Geometry: final body of the model. Coordinates: model frame, mm. A direction names the side the tool comes from. Give positions to 0.01 mm unless a question says otherwise; leave off trailing zeros. Write each loop counter-clockwise with the first axis right and the second up, starting at its lowest first coordinate (ties: lowest second). Pieces come first, ordered by that corner, then holes. Notation, with made-up numbers: (11, 27.25) - (18, 27.25) arc R25 cw to (18, 64.25) - close; hole circle Ø11 at (88, 84). An arc over 180 degrees is marked (long way). Return JSON: item names as keys, results as strings.
Autodesk Inventor part; units mm, degrees
ref_plane "YZ Plane" through (0, 0, 0) normal (1, 0, 0) x (0, 1, 0)
ref_plane "XZ Plane" through (0, 0, 0) normal (0, 1, 0) x (-1, 0, 0)
ref_plane "XY Plane" through (0, 0, 0) normal (0, 0, 1) x (1, 0, 0)
sketch "Sketch1" plane through (0, 0, 0) normal (0, 1, 0) x (-1, 0, 0)
  line L0 (1100, 990) -> (-1100, 990)
  line L1 (-1100, 990) -> (-1100, 0)
  line L2 (-1100, 0) -> (1100, 0)
  line L3 (1100, 0) -> (1100, 990)
  point P0 (0, 0)
  point P1 (0, 0)
  dimension "d0" = 2200
  dimension "d1" = 990
extrude "Extrusion1" add sketch "Sketch1" along normal blind 1020
sketch "Sketch2" plane through (1100, 0, 990) normal (1, 0, 0) x (0, 0, -1)
  line L0 (0, 0) -> (0, 1020)
  line L1 (0, 1020) -> (740, 1020)
  line L2 (740, 1020) -> (740, 600)
  line L3 (740, 600) -> (0, 600)
  line L4 (0, 600) -> (0, 1020)
  line L5 (990, 0) -> (990, 1020)
  point P0 (0, 600)
  dimension "d4" = 600
  dimension "d5" = 250
extrude "Extrusion2" cut sketch "Sketch2" against normal through all
sketch "Sketch3" plane through (1100, 600, 990) normal (0, 1, 0) x (1, 0, 0)
  line L0 (-2200, 0) -> (0, 0)
  line L1 (-2200, 740) -> (0, 740)
  line L2 (-1950, 0) -> (-250, 0)
  line L3 (-250, 0) -> (-250, 740)
  line L4 (-250, 740) -> (-1950, 740)
  line L5 (-1950, 740) -> (-1950, 0)
  line L6 (-2200, 0) -> (-2200, 740)
  point P0 (-1100, 990)
  point P1 (-1100, 0)
  point P2 (-1100, 0)
  point P3 (-1950, 740)
  point P4 (-250, 0)
  dimension "d8" = 250
extrude "Extrusion3" cut sketch "Sketch3" against normal blind 250 contours L5 L1 L3 L0
sketch "Sketch4" plane through (0, 0, 0) normal (0, -1, 0) x (1, 0, 0)
  line L0 (1100, 990) -> (1100, 0)
  line L1 (-1100, 990) -> (1100, 990)
  line L2 (-1100, 0) -> (-1100, 990)
  line L3 (1100, 0) -> (-1100, 0)
  line L4 (1000, 890) -> (1000, 100) construction
  line L5 (1000, 100) -> (-1000, 100) construction
  line L6 (-1000, 100) -> (-1000, 890) construction
  line L7 (-1000, 890) -> (1000, 890) construction
  circle A0 centre (-1000, 890) radius 25
  circle A1 centre (1000, 890) radius 25
  circle A2 centre (1000, 100) radius 25
  circle A3 centre (-1000, 100) radius 25
  point P0 (0, 0)
  dimension "d11" = 100
  dimension "d12" = 50
  dimension "d13" = 50
  dimension "d14" = 50
  dimension "d15" = 50
extrude "Extrusion4" cut sketch "Sketch4" against normal blind 100
properties part number "Divano Valdinoce"
Q1. Section query B-B, the plane x = 1000. Return the cut outline in (y, z).
Answer key:
{"outline": "(0, 75) - (100, 75) - (100, 0) - (1020, 0) - (1020, 250) - (600, 250) - (600, 990) - (100, 990) - (100, 915) - (0, 915) - (0, 865) - (100, 865) - (100, 125) - (0, 125) - close"}
Q2. Pin query (flat end, axial travel): P1, Ø8, axis at x = 73.5, y = 844.5, coming from the +Z side; P2, Ø4, axis at x = 125.5, z = 410, coming from the +Y side; P3, Ø10, axis at x = 552.5, y = 111, coming from the -Z side. Return the tip coordinate at first contact, or that it passes through.
Answer key:
{"P1": "stops at z = 250", "P2": "stops at y = 350", "P3": "stops at z = 0"}
Q3. Section query C-C, the plane y = 67.5. Return the cut outline in (x, z), plus the area to 3 significant figures.
Answer key:
{"outline": "circle Ø50 at (-1000, 100); circle Ø50 at (-1000, 890); circle Ø50 at (1000, 100); circle Ø50 at (1000, 890)", "area": "7,850 mm^2"}
Q4. Set-up query: faces 4 (the flat face through (-1100, 451, 378)), 5 (the flat face through (850, 477, 625)), 6 (the flat face through (1100, 451, 392)), 7 (the cylindrical face through (975.024, 49.3, 891.099)), 8 (the flat face through (-973, 600, 615)). Return all of +Z, -Z, +X, -X, +Y, -Y with unobstructed straight access to the full face (end or side cutting, diameter ignored); none if empty.
Answer key:
{"face 4": "+Z, -Z, -X, +Y, -Y", "face 5": "+Z, +Y", "face 6": "+Z, -Z, +X, +Y, -Y", "face 7": "-Y", "face 8": "+Z, +X, -X, +Y"}
Q5. Mould query, pull axis Z, two halves, no side actions, for faces 1 (the flat face through (-15, 291, 990)), 2 (the flat face through (1000, 0, 890)), 3 (the cylindrical face through (-1024.976, 49.3, 101.099)). Classes: pulls with the +Z half, pulls with the -Z half, needs draft (parallel to the pull), parting line crosses it, or undercut.
Answer key:
{"face 1": "pulls with the +Z half", "face 2": "needs draft", "face 3": "undercut"}
Q6. Material intervals for probe 1 along X at (y, z) = (457, 932); probe 2 along Y at (x, z) = (863, 670); probe 3 along Y at (x, z) = (-700.5, 819.5), sorted ascending. Write a range as [from, to].
Answer key:
{"probe 1": "x = [-1100, -850], [850, 1100]", "probe 2": "y = [100, 600]", "probe 3": "y = [100, 350]"}
Q7. Section query A-A, the plane z = 890. Return the cut outline in (x, y).
Answer key:
{"outline": "(-1100, 100) - (-1025, 100) - (-1025, 0) - (-975, 0) - (-975, 100) - (975, 100) - (975, 0) - (1025, 0) - (1025, 100) - (1100, 100) - (1100, 600) - (850, 600) - (850, 350) - (-850, 350) - (-850, 600) - (-1100, 600) - close"}
Q8. Section query D-D, the plane z = 100. Return the cut outline in (x, y).
Answer key:
{"outline": "(-1100, 100) - (-1025, 100) - (-1025, 0) - (-975, 0) - (-975, 100) - (975, 100) - (975, 0) - (1025, 0) - (1025, 100) - (1100, 100) - (1100, 1020) - (-1100, 1020) - close"}
